Autodesk Inventor part; units mm, degrees
ref_plane "YZ Plane" through (0, 0, 0) normal (1, 0, 0) x (0, 1, 0)
ref_plane "XZ Plane" through (0, 0, 0) normal (0, 1, 0) x (-1, 0, 0)
ref_plane "XY Plane" through (0, 0, 0) normal (0, 0, 1) x (1, 0, 0)
sketch "Sketch1" plane through (0, 0, 0) normal (0, 1, 0) x (-1, 0, 0)
  line L0 (82.171, 116.0061) -> (-97.829, 116.0061)
  line L1 (-97.829, 116.0061) -> (-97.829, -153.9939)
  line L2 (-97.829, -153.9939) -> (82.171, -153.9939)
  line L3 (81.171, 115.0061) -> (-96.829, 115.0061)
  line L4 (-96.829, 115.0061) -> (-96.829, -152.9939)
  line L5 (-96.829, -152.9939) -> (81.171, -152.9939)
  line L6 (81.171, 56.2728) -> (-8.329, -3.7272)
  line L7 (82.171, 55.7393) -> (-7.329, -4.2607)
  line L8 (82.171, -93.7272) -> (-7.329, -33.7272)
  line L9 (81.171, -94.2607) -> (-8.329, -34.2607)
  line L10 (81.171, 56.2728) -> (81.171, 115.0061)
  line L11 (82.171, -153.9939) -> (82.171, -93.7272)
  line L12 (82.171, 55.7393) -> (82.171, 116.0061)
  line L13 (-7.329, -4.2607) -> (-7.329, -33.7272)
  line L14 (-8.329, -3.7272) -> (-8.329, -34.2607)
  line L15 (81.171, -152.9939) -> (81.171, -94.2607)
  line L16 (-92.829, 111.0061) -> (77.171, 111.0061)
  line L17 (-92.829, 111.0061) -> (-92.829, -148.9939)
  line L18 (-92.829, -148.9939) -> (77.171, -148.9939)
  line L19 (-12.329, -1.5931) -> (-12.329, -36.3948)
  line L20 (77.171, 58.4069) -> (-12.329, -1.5931)
  line L21 (77.171, 111.0061) -> (77.171, 58.4069)
  line L22 (77.171, -96.3948) -> (77.171, -148.9939)
  line L23 (77.171, -96.3948) -> (-12.329, -36.3948)
  line L24 (67.171, 133.2815) -> (-82.829, 133.2815)
  line L25 (-82.829, 133.2815) -> (-82.829, 85.6394)
  line L26 (-82.829, 85.6394) -> (67.171, 85.6394)
  line L27 (67.171, 85.6394) -> (67.171, 133.2815)
  line L28 (91.8793, 101.0061) -> (59.7353, 101.0061)
  line L29 (59.7353, 101.0061) -> (59.7353, 70.7393)
  line L30 (59.7353, 70.7393) -> (91.8793, 70.7393)
  line L31 (91.8793, 70.7393) -> (91.8793, 101.0061)
  line L32 (74.0374, 40.9341) -> (7.2402, -3.8462)
  line L33 (56.8116, 66.6293) -> (-9.9856, 21.8491)
  line L34 (56.8116, 66.6293) -> (74.0374, 40.9341)
  line L35 (-9.9856, 21.8491) -> (7.2402, -3.8462)
  line L36 (-88.3298, 101.0061) -> (-103.1355, 101.0061)
  line L37 (-103.1355, 101.0061) -> (-103.1355, -3.9939)
  line L38 (-103.1355, -3.9939) -> (-88.3298, -3.9939)
  line L39 (-88.3298, -3.9939) -> (-88.3298, 101.0061)
  line L40 (-12.329, -18.9939) -> (-92.829, -18.9939)
  line L41 (67.171, -171.2694) -> (-82.829, -171.2694)
  line L42 (-82.829, -171.2694) -> (-82.829, -123.6273)
  line L43 (-82.829, -123.6273) -> (67.171, -123.6273)
  line L44 (67.171, -123.6273) -> (67.171, -171.2694)
  line L45 (91.8793, -138.9939) -> (59.7353, -138.9939)
  line L46 (59.7353, -138.9939) -> (59.7353, -108.7272)
  line L47 (59.7353, -108.7272) -> (91.8793, -108.7272)
  line L48 (91.8793, -108.7272) -> (91.8793, -138.9939)
  line L49 (74.0374, -78.922) -> (7.2402, -34.1417)
  line L50 (56.8116, -104.6172) -> (-9.9856, -59.837)
  line L51 (56.8116, -104.6172) -> (74.0374, -78.922)
  line L52 (-9.9856, -59.837) -> (7.2402, -34.1417)
  line L53 (-88.3298, -138.9939) -> (-103.1355, -138.9939)
  line L54 (-103.1355, -138.9939) -> (-103.1355, -33.9939)
  line L55 (-103.1355, -33.9939) -> (-88.3298, -33.9939)
  line L56 (-88.3298, -33.9939) -> (-88.3298, -138.9939)
  line L57 (79.671, -206.4141) -> (79.671, 178.4349)
  point P0 (0, 0)
  dimension "d0" = 270
  dimension "d3" = 1
  dimension "d4" = 1
  dimension "d5" = 1
  dimension "d17" = 5
  dimension "d18" = 29.4665
  dimension "d28" = 1
  dimension "d29" = 5
  dimension "d30" = 5
  dimension "d31" = 1
  dimension "d32" = 15
  dimension "d33" = 15
  dimension "d34" = 15
  dimension "d35" = 15
  dimension "d36" = 15
  dimension "d37" = 15
  dimension "d38" = 15
  dimension "d39" = 135
  dimension "d40" = 15
  dimension "d41" = 5
  dimension "d42" = 5
  dimension "d48" = 2.5
extrude "Extrusion1" add sketch "Sketch1" along normal blind 10 contours L12 L28 L10 L3 L57 L0 | L57 L3 L27 L0 | L12 L30 L10 L28 | L27 L3 L25 L0 | L12 L7 L57 L6 L10 L30 | L25 L3 L4 L36 L1 L0 | L7 L34 L6 L57 | L36 L4 L38 L1 | L7 L35 L6 L34 | L57 L9 L51 L8 | L8 L11 L47 L15 L9 L57 | L38 L4 L55 L1 | L7 L13 L8 L52 L9 L14 L6 L35 | L51 L9 L52 L8 | L55 L4 L53 L1 | L11 L45 L15 L47 | L53 L4 L5 L42 L2 L1 | L11 L2 L57 L5 L15 L45 | L57 L2 L44 L5 | L42 L5 L44 L2
extrude "Extrusion2" add sketch "Sketch1" along normal blind 1 contours L57 L28 L21 L16 L27 L3 | L3 L10 L28 L57 | L10 L30 L57 L28 | L27 L16 L25 L3 | L57 L30 L21 L28 | L10 L6 L57 L30 | L25 L16 L17 L36 L4 L3 | L57 L6 L34 L20 L21 L30 | L36 L17 L38 L4 | L6 L35 L20 L34 | L57 L47 L22 L23 L51 L9 | L9 L15 L47 L57 | L38 L17 L55 L4 | L6 L14 L9 L52 L23 L19 L20 L35 | L51 L23 L52 L9 | L57 L45 L22 L47 | L47 L15 L45 L57 | L55 L17 L53 L4 | L57 L5 L44 L18 L22 L45 | L45 L15 L5 L57 | L53 L17 L18 L42 L5 L4 | L5 L42 L18 L44
extrude "Extrusion3" cut sketch "Sketch1" along normal blind 7.5 contours L28 L31 L30 L12 | L12 L30 L10 L28 | L27 L3 L25 L0 | L0 L25 L24 L27 | L10 L30 L57 L28 | L27 L16 L25 L3 | L57 L30 L21 L28 | L27 L28 L29 L26 L25 L16 | L21 L30 L29 L26 L27 L28 | L36 L4 L38 L1 | L1 L38 L37 L36 | L27 L26 L29 L28 | L34 L32 L35 L7 | L7 L35 L6 L34 | L36 L17 L38 L4 | L6 L35 L20 L34 | L51 L9 L52 L8 | L8 L52 L49 L51 | L55 L4 L53 L1 | L1 L53 L54 L55 | L36 L39 L38 L17 | L20 L35 L33 L34 | L47 L48 L45 L11 | L11 L45 L15 L47 | L51 L23 L52 L9 | L57 L45 L22 L47 | L47 L15 L45 L57 | L55 L17 L53 L4 | L51 L50 L52 L23 | L22 L45 L44 L43 L46 L47 | L55 L56 L53 L17 | L42 L5 L44 L2 | L2 L44 L41 L42 | L45 L46 L43 L44 | L44 L18 L42 L43 L46 L45 | L5 L42 L18 L44
fillet "Fillet1" radius 1 15 edges at (2.9857, 1, -0.1451) (8.329, 1, -18.9939) (-81.171, 1, -101.4939) (-74.171, 1, -152.9939) (-81.171, 1, -145.9939) (-75.1629, 1, 52.2451) (-81.171, 1, 63.5061) (-81.171, 1, 108.0061) (-74.171, 1, 115.0061) (89.829, 1, 115.0061) (96.829, 1, 108.0061) (96.829, 1, -18.9939) (96.829, 1, -145.9939) (2.9857, 1, -37.8428) (89.829, 1, -152.9939)
sketch "Sketch2" plane through (0, 0, 0) normal (0, -1, 0) x (1, 0, 0)
  line L0 (135.8296, -18.9939) -> (-115.0378, -18.9939)
  line L1 (-115.0378, -18.9939) -> (-115.0378, 152.8468)
  line L2 (-115.0378, 152.8468) -> (135.8296, 152.8468)
  line L3 (135.8296, 152.8468) -> (135.8296, -18.9939)
  line L4 (-115.0378, -18.9939) -> (154.388, -18.9939)
  line L5 (154.388, -18.9939) -> (154.388, -183.4288)
  line L6 (154.388, -183.4288) -> (-115.0378, -183.4288)
  line L7 (-115.0378, -183.4288) -> (-115.0378, -18.9939)
  point P0 (0, 0)
extrude "Extrusion4" cut sketch "Sketch2" against normal blind 100 contours L0 L1 L2 L3 keep common part
sketch "Sketch4" plane through (97.829, 0, -18.9939) normal (0, 0, -1) x (-1, 0, 0)
  line L0 (0, 0) -> (5, 0)
  line L1 (5, 0) -> (5, 7.5)
  line L2 (5, 7.5) -> (0, 7.5)
  line L3 (0, 7.5) -> (0, 0)
  line L4 (90.5, 0) -> (85.5, 0)
  line L5 (85.5, 0) -> (85.5, 7.5)
  line L6 (85.5, 7.5) -> (90.5, 7.5)
  line L7 (90.5, 7.5) -> (90.5, 0)
  point P0 (97.829, 0)
  dimension "d55" = 5
  dimension "d56" = 5
  dimension "d57" = 7.5
  dimension "d58" = 7.5
extrude "Extrusion6" add sketch "Sketch4" against normal blind 1
properties part number "Female"
Model file for the job. Use its own axes, mm. A direction names the side the tool comes from. Round coordinates to 2 decimals unless told otherwise and drop trailing zeros. Loops run counter-clockwise (first coordinate to the right, second up) from the corner with the lowest first, then second, coordinate; pieces in that order, holes last. Notation, with made-up numbers: (18, 72) -> (69, 72) arc R21 cw to (69, 105) -> close; hole circle Ø8 at (17, 44.5). An arc over 180 degrees is marked (long way). Answer as CSV lines item,"result". Start each with the question number.
1) Probe line 1 along X through (y, z) = (2.75, -5.5); line 2 along X through (y, z) = (8, 57); line 3 along Z through (x, y) = (10, 6.25). List the from-to ranges inside material, lowest first.
2) Mould opens along X. For faces 6 (the face through (-67.171, 2.6, 115.2)), 7 (the face through (7.329, 5, -12)), 8 (the face through (8, 0, -6)) say: +X half, -X half, draft (parallel to the pull), parting line (faces both ways), or undercut.
3) Slice it at A-A (z = 105). List the corners of the cut face in (x, y).
4) Slice it at B-B (y = 3.5). State how many separate pieces and enclosed holes the cut face has, plus the area to 3 significant figures.
5) Slice it at C-C (x = -23.5). List the corners of the cut face in (y, z).
6) Slice it at D-D (z = 43). List the corners of the cut face in (x, y), plus the area to 3 significant figures.
7) Tool access for faces 1 (the face through (-2.444, 2.621, 3.308)), 2 (the face through (97, 3, 101.006)), 3 (the face through (10, 4, -17.994)), 4 (the face through (97, 2, -3.994)), 5 (the face through (92, 1, 112)): list every direction of +Z, -Z, +X, -X, +Y, -Y with a clear straight run to the whole face (end or side of a thin tool).
8) Pin check, flat tips, straight feed: P1, Ø0.5, axis at y = 0.5, z = 64, coming from the +X side; P2, Ø0.8, axis at x = -81.5, z = 85.5, coming from the -Y side; P3, Ø1.5, axis at y = 5.5, z = 67.5, coming from the +X side. Stop position of each tip, or through.
Filled in:
1,line 1,"x = 7.33 to 8.33, 96.83 to 97.83"
1,line 2,"x = -82.17 to -81.17, 96.83 to 97.83"
1,line 3,"z = -18.99 to -17.99"
2,face 6,"undercut"
2,face 7,"-X half"
2,face 8,"draft"
3,outline,"(-82.17, 0) -> (-77.17, 0) -> (-77.17, 1) -> (-80.17, 1) arc R1 cw to (-81.17, 2) -> (-81.17, 10) -> (-82.17, 10) -> close; (92.83, 0) -> (97.83, 0) -> (97.83, 10) -> (96.83, 10) -> (96.83, 2) arc R1 cw to (95.83, 1) -> (92.83, 1) -> close"
4,separate pieces,"5"
4,enclosed holes,"0"
4,area,"138 mm2"
5,outline,"(7.5, 16.41) -> (10, 16.41) -> (10, 17.61) -> (7.5, 17.61) -> close; (7.5, 115.01) -> (10, 115.01) -> (10, 116.01) -> (7.5, 116.01) -> close"
6,outline,"(-63.17, 7.5) -> (-61.37, 7.5) -> (-61.37, 10) -> (-63.17, 10) -> close; (96.83, 7.5) -> (97.83, 7.5) -> (97.83, 10) -> (96.83, 10) -> close"
6,area,"6.99 mm2"
7,face 1,"+Z, -X, -Y"
7,face 2,"+X, -X, -Y"
7,face 3,"+Z, +Y"
7,face 4,"+X, -Y"
7,face 5,"+Y"
8,P1,"stops at x = -77.17"
8,P2,"stops at y = 7.5"
8,P3,"stops at x = -81.17"
